Source: CAD feature listing. Evaluate the final solid. Frame: model axes, mm. A direction names the side the tool comes from. Give positions to 0.01 mm unless a question says otherwise; leave off trailing zeros. Order: outer loops, then holes, each group sorted by start corner. A loop starts at its lowest first (then second) coordinate and runs counter-clockwise, first axis right, second up. Notation, with made-up numbers: M 20.5,59 L 59.5,59 A10 ccw 59.5,71 Z; hole C 17.25,-6 d9. An arc over 180 degrees is marked long. Answer in a Markdown table with one row per item. Add a question column.
(1) Section query C-C, the plane z = 4.5. Return loops of the section in (x, y).
(2) Section query A-A, the plane y = 2.55. Return loops of the section in (x, z), plus the area to 3 significant figures.
(3) Section query D-D, the plane y = 3.75. Return loops of the section in (x, z), plus the area to 3 significant figures.
(4) Mould query, pull axis Z, two halves, no side actions, for faces 6 (the face through (-71.355, 3, 5)), 7 (the face through (-68, 0.9, 5)), 8 (the face through (-70, 2, 9)), 9 (the face through (-67.44, 2.43, 9.65)). Classes: pulls with the +Z half, pulls with the -Z half, needs draft (parallel to the pull), parting line crosses it, or undercut.
(5) Section query B-B, the plane x = -70.75. Return loops of the section in (y, z).
(6) Set-up query: faces 1 (the face through (-69.9, 0.918, 0.5)), 2 (the face through (-74, 2, 0)), 3 (the face through (-70, 2, 1)), 4 (the face through (-67.155, 2, 5)), 5 (the face through (-68, 3.918, 5)). Return all of +Z, -Z, +X, -X, +Y, -Y with unobstructed straight access to the full face (end or side cutting, diameter ignored); none if empty.
(7) Pin query (flat end, axial travel): P1, Ø1, axis at x = -67.5, z = 4.5, coming from the -Y side; P2, Ø4.5, axis at x = -68.5, z = 5.5, coming from the +Y side. Return the tip coordinate at first contact, or that it passes through.
(8) Material intervals for line 1 along X through (y, z) = (2.75, 2.75); line 2 along Y through (x, z) = (-68.25, 0.5); line 3 along X through (y, z) = (3.5, 5.5), sorted ascending.
from build123d import *

# Parameters (mm, degrees)
SKETCH_1_R            = 5
EXTRUDE_1_DEPTH       = 10
SKETCH_9_W            = 7.120641766
SKETCH_9_H            = 4.534999238
EXTRUDE_6_DEPTH       = 1
SKETCH_11_W           = 1.257653538
SKETCH_11_H           = 9
EXTRUDE_7_DEPTH       = 4.5
EXTRUDE_8_DEPTH       = 6
FILLET_8_R            = 1
FILLET_9_R            = 1
CUT_EXTRUDE_1_DEPTH   = 10
SKETCH_14_W           = 1
SKETCH_14_H           = 3
EXTRUDE_9_DEPTH       = 3.122043073
SKETCH_15_W           = 1
SKETCH_15_H           = 3
EXTRUDE_10_DEPTH      = 4
EXTRUDE_11_DEPTH      = 0.2
EXTRUDE_11_DEPTH_BACK = 1.043632387
SKETCH_16_W           = 9.952294967
SKETCH_16_H           = 3.01746433
FILLET_11_R           = 1
FILLET_12_R           = 1
FILLET_13_R           = 1
FILLET_14_R           = 1


with BuildPart() as part:
    # Sketch 1 → Extrude 1 (new body)
    with BuildSketch(Plane(origin=(0.382706605, 0, 0), x_dir=(1, 0, 0), z_dir=(0, 0, 1))):
        with Locations((-75.594417438, 2.55)):
            Circle(SKETCH_1_R)
    extrude(amount=EXTRUDE_1_DEPTH)

    # Sketch 9 → Extrude 6 (add)
    with BuildSketch(Plane(origin=(6.127831546, 0, 9), x_dir=(1, 0, 0), z_dir=(0, 0, 1))):
        with Locations((-75.644850643, 2.267499619)):
            Rectangle(SKETCH_9_W, SKETCH_9_H)
    extrude(amount=EXTRUDE_6_DEPTH)



with BuildPart() as body_2:
    # Sketch 11 → Extrude 7 (new body)
    with BuildSketch(Plane(origin=(9.574526933, 4.534999238, 0.48426017), x_dir=(1, 0, 0), z_dir=(0, 1, 0))):
        with Locations((-76.184774061, -4.5)):
            Rectangle(SKETCH_11_W, SKETCH_11_H)
    extrude(amount=-EXTRUDE_7_DEPTH)


with BuildPart() as part_1:
    add(part.part)

    add(body_2.part)  # Extrude 8 merges body 2
    # Sketch 12 → Extrude 8 (add)
    with BuildSketch(Plane.ZY.offset(67.239073897)):
        Polygon((0.48426017, 4.534999238), (0.48426017, 0), (1.483647509, 0.034999238), (1.483647509, 4.534999238), align=None)
    extrude(amount=EXTRUDE_8_DEPTH)

    # Fillet 8
    fillet_8_edges = [part_1.edges().sort_by_distance(p)[0] for p in [
        (-65.981420359, 2.284999238, 0.48426017),
    ]]
    fillet(fillet_8_edges, radius=FILLET_8_R)

    # Fillet 9
    fillet_9_edges = [part_1.edges().sort_by_distance(p)[0] for p in [
        (-65.956698214, 2.267499619, 10),
    ]]
    fillet(fillet_9_edges, radius=FILLET_9_R - 0.0001)  # a hair under: the kernel refuses the full size

    # Sketch 13 → Cut-Extrude 1 (cut)
    with BuildSketch(Plane(origin=(0, 0, 0), x_dir=(-1, 0, 0), z_dir=(0, 0, -1))):
        with BuildLine():
            Line((71.355365605, 5.732546384), (71.355365605, -0.632546384))
            ThreePointArc((71.355365605, -0.632546384), (70.211710833, 2.55), (71.355365605, 5.732546384))
        make_face()
    extrude(amount=-CUT_EXTRUDE_1_DEPTH, mode=Mode.SUBTRACT)


with BuildPart() as body_2_2:
    # of the pieces the cut leaves, the one that is kept (cut_extrude_1_keep)
    add(part_1.part.solids().sort_by_distance((-71.355365605, 5.732546384, 0))[0])

    # Sketch 14 → Extrude 9 (add)
    with BuildSketch(Plane(origin=(-71.355365605, 0, 0), x_dir=(0, 0, -1), z_dir=(1, 0, 0))):
        with Locations((-9.5, 2.417510407)):
            Rectangle(SKETCH_14_W, SKETCH_14_H)
    extrude(amount=EXTRUDE_9_DEPTH)

    # Sketch 15 → Extrude 10 (add)
    with BuildSketch(Plane(origin=(-71.355365605, 0, 0), x_dir=(0, 0, -1), z_dir=(1, 0, 0))):
        with Locations((-0.5, 2.417510407)):
            Rectangle(SKETCH_15_W, SKETCH_15_H)
    extrude(amount=EXTRUDE_10_DEPTH)

    # Sketch 16 → Extrude 11 (add, two sides: drawn at the far end of the back side and taken through both)
    with BuildSketch(Plane(origin=(-67.355365605, 0, 0), x_dir=(0, 0, -1), z_dir=(1, 0, 0)).offset(-EXTRUDE_11_DEPTH_BACK)):
        with Locations((-4.976147484, 2.408778242)):
            Rectangle(SKETCH_16_W, SKETCH_16_H)
    extrude(amount=EXTRUDE_11_DEPTH + EXTRUDE_11_DEPTH_BACK)

    # Fillet 11
    fillet_11_edges = [body_2_2.edges().sort_by_distance(p)[0] for p in [
        (-67.155365605, 2.408778242, 0),
    ]]
    fillet(fillet_11_edges, radius=FILLET_11_R)

    # Fillet 12
    fillet_12_edges = [body_2_2.edges().sort_by_distance(p)[0] for p in [
        (-67.155365605, 2.408778242, 9.952294967),
    ]]
    fillet(fillet_12_edges, radius=FILLET_12_R)

    # Fillet 13
    fillet_13_edges = [body_2_2.edges().sort_by_distance(p)[0] for p in [
        (-71.355365605, 5.732546384, 5),
    ]]
    fillet(fillet_13_edges, radius=FILLET_13_R)

    # Fillet 14
    fillet_14_edges = [body_2_2.edges().sort_by_distance(p)[0] for p in [
        (-71.355365605, -0.632546384, 5),
    ]]
    fillet(fillet_14_edges, radius=FILLET_14_R)


solid = body_2_2.part
Values follow:
| question | item | result |
|---|---|---|
| 1 | outline | M -71.64,-0.95 A1 ccw -71.36,-0.25 L -71.36,5.35 A1 ccw -71.64,6.05 A5 ccw long Z; M -68.4,0.9 L -67.16,0.9 L -67.16,3.92 L -68.4,3.92 Z |
| 2 | outline | M -80.21,0 L -68.16,0 A1 ccw -67.16,1 L -67.16,8.95 A1 ccw -68.16,9.95 L -68.23,9.95 L -68.23,10 L -80.21,10 Z; hole M -71.36,1 L -68.4,1 L -68.4,9 L -71.36,9 Z |
| 2 | area | 106 mm² |
| 3 | outline | M -80.07,0 L -68.16,0 A1 ccw -67.16,1 L -67.16,8.95 A1 ccw -68.16,9.95 L -68.23,9.95 L -68.23,10 L -80.07,10 Z; hole M -71.36,1 L -68.4,1 L -68.4,9 L -71.36,9 Z |
| 3 | area | 105 mm² |
| 4 | face 6 | undercut |
| 4 | face 7 | needs draft |
| 4 | face 8 | undercut |
| 4 | face 9 | pulls with the +Z half |
| 5 | outline | M 0.92,0 L 3.92,0 L 3.92,1 L 0.92,1 Z; M 0.92,9 L 3.92,9 L 3.92,10 L 0.92,10 Z |
| 6 | face 1 | +Z, -Z, -Y |
| 6 | face 2 | -Z, +X, -X, +Y, -Y |
| 6 | face 3 | +Y, -Y |
| 6 | face 4 | +Z, -Z, +X, +Y, -Y |
| 6 | face 5 | +Z, -Z, +X, +Y |
| 7 | P1 | stops at y = 0.9 |
| 7 | P2 | stops at y = 3.92 |
| 8 | line 1 | x = -80.21 to -71.36, -68.4 to -67.16 |
| 8 | line 2 | y = 0.9 to 3.92 |
| 8 | line 3 | x = -80.12 to -71.36, -68.4 to -67.16 |
